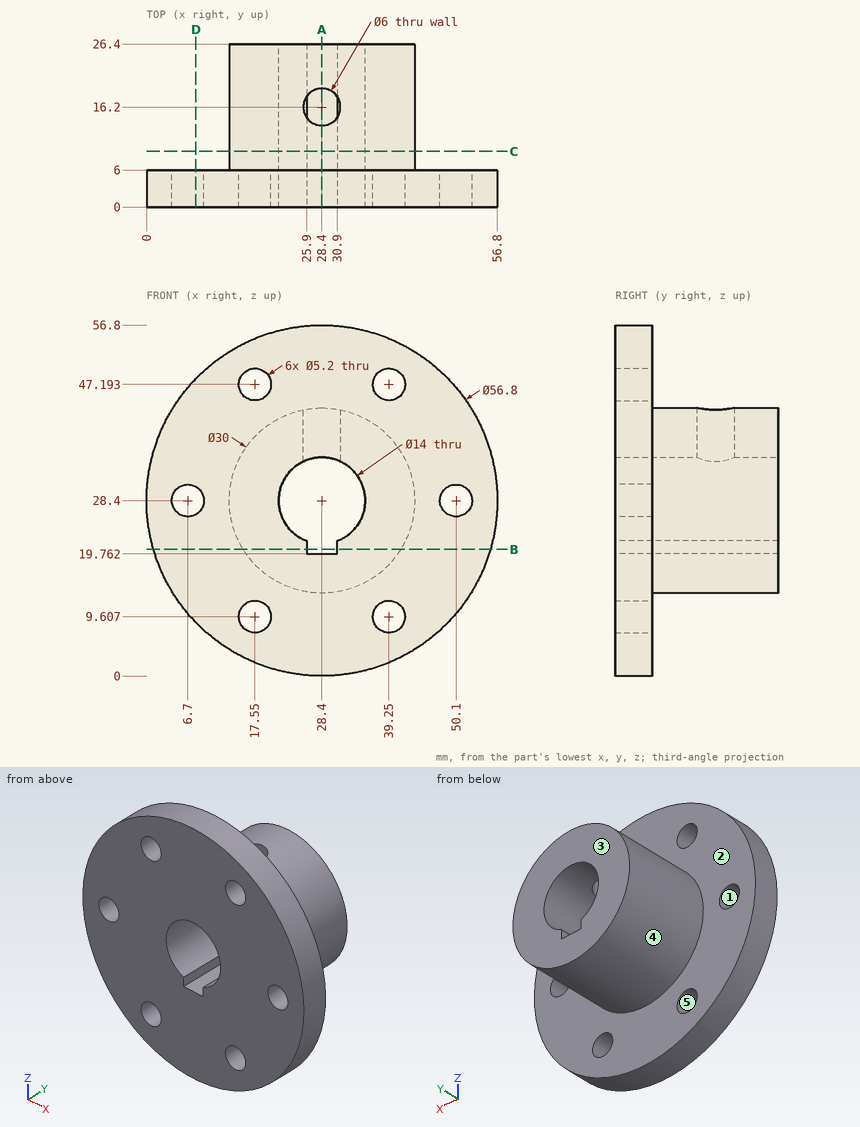
Job drawing, mm, ordinate dimensions from the low corner. One solid piece. A direction names the side the tool comes from. Give positions to 0.01 mm unless a question says otherwise; leave off trailing zeros. Order: outer loops, then holes, each group sorted by start corner. A loop starts at its lowest first (then second) coordinate and runs counter-clockwise, first axis right, second up. Notation, with made-up numbers: M 12,4.25 L 43,4.25 A11 cw 43,12.25 Z; hole C -25.5,55 d3. An arc over 180 degrees is marked long. Put each result on its own line as item: value. Start each with the question number.
(1) Pull direction Z, two halves, no side cores. Call the marked faces 3, 4 and 5: released by +Z, released by -Z, zero draft, split by the parting line, or undercut.
(2) Band-saw the part on C-C on y = 9. Give the cut face in (x, z).
(3) Tool access for the marked faces 1 and 2: list every direction of +Z, -Z, +X, -X, +Y, -Y with a clear straight run to the whole face (end or side of a thin tool).
(4) Band-saw the part on B-B on z = 20.5. Give the cut face in (x, y).
(5) Band-saw the part on A-A on x = 28.4. Give the cut face in (y, z), then the cut area to 3 significant figures.
(6) Pin check, flat tips, straight feed: pin 1 Ø12 at (x, y) = (12, 9.5) entering from -Z (1 decimal); pin 2 Ø3 at (x, y) = (34, 9.5) entering from -Z; pin 3 Ø3 at (x, z) = (50.1, 28.4) entering from +Y (3 decimals); pin 4 Ø1.1 at (y, z) = (14, 20.5) entering from -X (1 decimal). Stop position of each tip, or through.
(7) Band-saw the part on D-D on x = 8. Give the cut face in (y, z).
(8) Drill centre lines: L1, parallel to X at y = 3.95, z = 28.4; L2, parallel to X at y = 18, z = 28.4; L3, parallel to Y at x = 28.4, z = 40.5. Where is each one in solid material? Low to high. Write a range as [from, to].
Results below:
1. face 3: zero draft
1. face 4: split by the parting line
1. face 5: undercut
2. outline: C 28.4,28.4 d30; hole M 25.9,19.76 L 30.9,19.76 L 30.9,21.86 A7 ccw long 25.9,21.86 Z
3. face 1: +Y, -Y
3. face 2: +Y
4. outline: M 1.12,0 L 25.9,0 L 25.9,26.4 L 15.65,26.4 L 15.65,6 L 1.12,6 Z; M 30.9,0 L 55.68,0 L 55.68,6 L 41.15,6 L 41.15,26.4 L 30.9,26.4 Z
5. outline: M 0,0 L 6,0 L 6,13.4 L 26.4,13.4 L 26.4,19.76 L 0,19.76 Z; M 0,35.4 L 13.2,35.4 L 13.2,43.4 L 6,43.4 L 6,56.8 L 0,56.8 Z; M 19.2,35.4 L 26.4,35.4 L 26.4,43.4 L 19.2,43.4 Z
5. area: 492 mm2
6. pin 1: stops at z = 2.4
6. pin 2: stops at z = 13.97
6. pin 3: passes through
6. pin 4: stops at x = 15.3
7. outline: M 0,8.64 L 6,8.64 L 6,26.15 L 0,26.15 Z; M 0,30.65 L 6,30.65 L 6,48.16 L 0,48.16 Z
8. L1: x = [0, 4.1], [9.3, 21.4], [35.4, 47.5], [52.7, 56.8]
8. L2: x = [13.4, 21.4], [35.4, 43.4]
8. L3: y = [0, 13.2], [19.2, 26.4]
